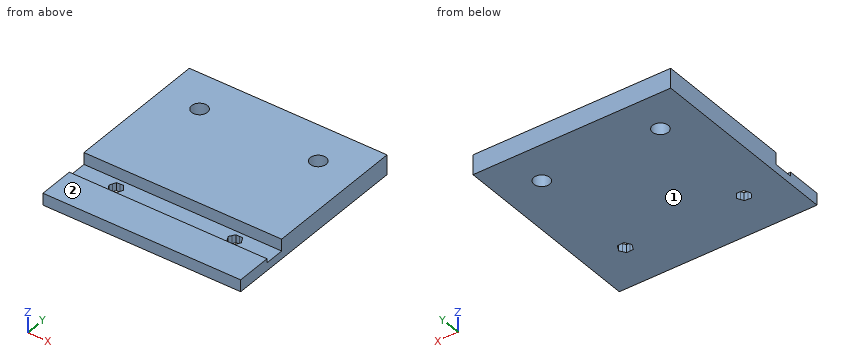
```python
from build123d import *

# Parameters (mm, degrees)
F0_W     = 100
F0_H     = 100
F1_DEPTH = 4
F2_W     = 100
F2_H     = 72
F2_H_2   = 18
F3_DEPTH = 2
F4_W     = 100
F4_H     = 72
F5_DEPTH = 4
F6_R     = 4
F7_DEPTH = 25


with BuildPart() as f1:
    # F0 (on Top) → F1 (new body)
    with BuildSketch(Plane.XY):
        Rectangle(F0_W, F0_H)
    extrude(amount=F1_DEPTH)

    # F2 (on face) → F3 (join)
    with BuildSketch(Plane.XY.offset(4)):
        with Locations((0, 14)):
            Rectangle(F2_W, F2_H)
        with Locations((0, -41)):
            Rectangle(F2_W, F2_H_2)
    extrude(amount=F3_DEPTH)

    # F4 (on face) → F5 (join)
    with BuildSketch(Plane.XY.offset(6)):
        with Locations((0, 14)):
            Rectangle(F4_W, F4_H)
    extrude(amount=F5_DEPTH)

    # F6 (on face) → F7 (cut)
    with BuildSketch(Plane.XY.offset(10)):
        with Locations((30, 30)):
            Circle(F6_R)
        with Locations((-30, 30)):
            Circle(F6_R)
        with BuildLine():
            ThreePointArc((-27.2789726301, -28.3521687498), (-27.0705732549, -27.7357198631), (-27, -27.0888358355))
            ThreePointArc((-27, -27.0888358355), (-27.1396000204, -26.1843404199), (-27.5454079712, -25.3640233899))
            ThreePointArc((-27.5454079712, -25.3640233899), (-28.7366669855, -24.3678085121), (-30.2664349753, -24.1006905237))
            ThreePointArc((-30.2664349753, -24.1006905237), (-31.7248121898, -24.634243627), (-32.721027317, -25.8255028072))
            ThreePointArc((-32.721027317, -25.8255028072), (-32.9881452887, -27.3552710687), (-32.4545920728, -28.8136482183))
            ThreePointArc((-32.4545920728, -28.8136482183), (-31.2633329265, -29.8098631997), (-29.7335647552, -30.0769811231))
            ThreePointArc((-29.7335647552, -30.0769811231), (-28.2751876481, -29.54342793), (-27.2789726301, -28.3521687498))
        make_face()
        with BuildLine():
            ThreePointArc((-27.5454079712, -25.3640233899), (-27.1396000204, -26.1843404199), (-27, -27.0888358355))
            ThreePointArc((-27, -27.0888358355), (-27.0705732549, -27.7357198631), (-27.2789726301, -28.3521687498))
            Line((-27.2789726301, -28.3521687498), (-26.5495870229, -26.7811829673))
            Line((-26.5495870229, -26.7811829673), (-27.5454079712, -25.3640233899))
        make_face()
        with BuildLine():
            ThreePointArc((-30.2664349753, -24.1006905237), (-28.7366669855, -24.3678085121), (-27.5454079712, -25.3640233899))
            Line((-27.5454079712, -25.3640233899), (-28.5412287108, -23.9468641096))
            Line((-28.5412287108, -23.9468641096), (-30.2664349753, -24.1006905237))
        make_face()
        with BuildLine():
            Line((-28.0083583121, -29.9231546931), (-27.2789726301, -28.3521687498))
            ThreePointArc((-27.2789726301, -28.3521687498), (-28.2751876481, -29.54342793), (-29.7335647552, -30.0769811231))
            Line((-29.7335647552, -30.0769811231), (-28.0083583121, -29.9231546931))
        make_face()
        with BuildLine():
            ThreePointArc((-32.721027317, -25.8255028072), (-31.7248121898, -24.634243627), (-30.2664349753, -24.1006905237))
            Line((-30.2664349753, -24.1006905237), (-31.9916416879, -24.2545169778))
            Line((-31.9916416879, -24.2545169778), (-32.721027317, -25.8255028072))
        make_face()
        with BuildLine():
            Line((-31.4587712892, -30.2308075613), (-29.7335647552, -30.0769811231))
            ThreePointArc((-29.7335647552, -30.0769811231), (-31.2633329265, -29.8098631997), (-32.4545920728, -28.8136482183))
            Line((-32.4545920728, -28.8136482183), (-31.4587712892, -30.2308075613))
        make_face()
        with BuildLine():
            ThreePointArc((-32.4545920728, -28.8136482183), (-32.9881452887, -27.3552710687), (-32.721027317, -25.8255028072))
            Line((-32.721027317, -25.8255028072), (-33.4504129771, -27.3964887036))
            Line((-33.4504129771, -27.3964887036), (-32.4545920728, -28.8136482183))
        make_face()
        with BuildLine():
            ThreePointArc((32.5153308801, -28.7239650037), (32.876281683, -27.9416451078), (33, -27.089))
            ThreePointArc((33, -27.089), (32.9172554923, -26.3892712006), (32.6735864049, -25.7281415445))
            ThreePointArc((32.6735864049, -25.7281415445), (31.6349646218, -24.5736688716), (30.1582554561, -24.0931770395))
            ThreePointArc((30.1582554561, -24.0931770395), (28.6391417683, -24.4154134812), (27.4846689431, -25.4540352683))
            ThreePointArc((27.4846689431, -25.4540352683), (27.0041770385, -26.9307445628), (27.3264135035, -28.4498582753))
            ThreePointArc((27.3264135035, -28.4498582753), (28.365035239, -29.6043310379), (29.8417444141, -30.0848229536))
            ThreePointArc((29.8417444141, -30.0848229536), (31.3608580292, -29.7625866218), (32.5153308801, -28.7239650037))
        make_face()
        with BuildLine():
            ThreePointArc((32.6735864049, -25.7281415445), (32.9172554923, -26.3892712006), (33, -27.089))
            ThreePointArc((33, -27.089), (32.876281683, -27.9416451078), (32.5153308801, -28.7239650037))
            Line((32.5153308801, -28.7239650037), (33.4592783853, -27.2717376616))
            Line((33.4592783853, -27.2717376616), (32.6735864049, -25.7281415445))
        make_face()
        with BuildLine():
            ThreePointArc((30.1582554561, -24.0931770395), (31.6349646218, -24.5736688716), (32.6735864049, -25.7281415445))
            Line((32.6735864049, -25.7281415445), (31.8878946499, -24.1845458704))
            Line((31.8878946499, -24.1845458704), (30.1582554561, -24.0931770395))
        make_face()
        with BuildLine():
            Line((31.5713837355, -30.1761917913), (32.5153308801, -28.7239650037))
            ThreePointArc((32.5153308801, -28.7239650037), (31.3608580292, -29.7625866218), (29.8417444141, -30.0848229536))
            Line((29.8417444141, -30.0848229536), (31.5713837355, -30.1761917913))
        make_face()
        with BuildLine():
            ThreePointArc((27.4846689431, -25.4540352683), (28.6391417683, -24.4154134812), (30.1582554561, -24.0931770395))
            Line((30.1582554561, -24.0931770395), (28.4286162645, -24.0018082087))
            Line((28.4286162645, -24.0018082087), (27.4846689431, -25.4540352683))
        make_face()
        with BuildLine():
            Line((28.1121053501, -29.9934541296), (29.8417444141, -30.0848229536))
            ThreePointArc((29.8417444141, -30.0848229536), (28.365035239, -29.6043310379), (27.3264135035, -28.4498582753))
            Line((27.3264135035, -28.4498582753), (28.1121053501, -29.9934541296))
        make_face()
        with BuildLine():
            ThreePointArc((27.3264135035, -28.4498582753), (27.0041770385, -26.9307445628), (27.4846689431, -25.4540352683))
            Line((27.4846689431, -25.4540352683), (26.5407216147, -26.9062623384))
            Line((26.5407216147, -26.9062623384), (27.3264135035, -28.4498582753))
        make_face()
    extrude(amount=-F7_DEPTH, mode=Mode.SUBTRACT)


solid = f1.part
```
Input: part model. Units: mm. Frame: model coordinates. Face numbers are marked on the shaded views. A direction names the side the tool comes from. Coordinates: 2 decimals unless noted, no trailing zeros. Order: outer loops, then holes, each group sorted by start corner. A loop starts at its lowest first (then second) coordinate and runs counter-clockwise, first axis right, second up. Notation, with made-up numbers: (-33, 43.25) - (-26, 43.25) arc R21 cw to (-26, 67.25) - close; hole circle Ø7 at (77, 84.25). An arc over 180 degrees is marked (long way). Put each result on its own line as item: value.
1. Reachability of the marked faces 1 and 2 from +Z, -Z, +X, -X, +Y, -Y: full face, straight path, thin tool, end or side. Return the list, or none.
Report:
face 1: -Z, +X, -X, +Y, -Y
face 2: +Z, +X, -X, -Y
2. Cut plane A-A on y = 30. Return the cut outline in (x, z).
Report:
outline: (-50, 0) - (-34, 0) - (-34, 10) - (-50, 10) - close; (-26, 0) - (26, 0) - (26, 10) - (-26, 10) - close; (34, 0) - (50, 0) - (50, 10) - (34, 10) - close
3. Cut plane D-D on y = -41.5. Return the cut outline in (x, z), then the cut area to 3 significant figures.
Report:
outline: (-50, 0) - (50, 0) - (50, 6) - (-50, 6) - close
area: 600 mm2
4. Contact query for flat-ended pins moving along their axis: pin 1 Ø2 at (x, y) = (-35, 16) entering from -Z; pin 2 Ø20 at (x, y) = (9, -43.5) entering from +Z; pin 3 Ø5 at (x, y) = (-6.5, -25) entering from +Z. Output: stop coordinate, or through.
Report:
pin 1: stops at z = 0
pin 2: stops at z = 6
pin 3: stops at z = 4
5. Cut plane B-B on x = 8.5. Return the cut outline in (y, z).
Report:
outline: (-50, 0) - (50, 0) - (50, 10) - (-22, 10) - (-22, 4) - (-32, 4) - (-32, 6) - (-50, 6) - close
6. Line query: line 1 along Y through (x, z) = (30, 3.5); line 2 along Y through (x, z) = (30, 7.25); line 3 along Y through (x, z) = (-44, 5.5). Output: solid intervals per line, ascending.
Report:
line 1: y = -50 to -30.09, -24.08 to 26, 34 to 50
line 2: y = -22 to 26, 34 to 50
line 3: y = -50 to -32, -22 to 50
7. Cut plane C-C on z = 8. Return the cut outline in (x, y), then the cut area to 3 significant figures.
Report:
outline: (-50, -22) - (50, -22) - (50, 50) - (-50, 50) - close; hole circle Ø8 at (-30, 30); hole circle Ø8 at (30, 30)
area: 7,100 mm2
